Design review of the part built by this model. Coordinates are the model's own, in mm. A direction names the side the tool comes from. Give positions to 0.01 mm unless a question says otherwise; leave off trailing zeros. Order: outer loops, then holes, each group sorted by start corner. A loop starts at its lowest first (then second) coordinate and runs counter-clockwise, first axis right, second up. Notation, with made-up numbers: (55, 53.5) -> (104, 53.5) arc R14 cw to (104, 70.5) -> close; hole circle Ø4 at (22.25, 15). An arc over 180 degrees is marked (long way). One line per item, written item: value.
from build123d import *

# Parameters (mm, degrees)
SKETCH1_W            = 279.4
SKETCH1_H            = 101.6
BOSS_EXTRUDE1_DEPTH  = 6.35
SKETCH2_R            = 13.97
BOSS_EXTRUDE3_DEPTH  = 5.55625
SKETCH9_R            = 11.1125
CUT_EXTRUDE4_DEPTH   = 4.445
CUT_EXTRUDE5_START   = -5.55625
SKETCH10_R           = 11.1125
CUT_EXTRUDE5_DEPTH   = 5.55625
SKETCH11_R           = 7.9375
CUT_EXTRUDE6_DEPTH   = 285.078633923
SKETCH12_R           = 6.35
CUT_EXTRUDE7_DEPTH   = 285.051619429
SKETCH22_W           = 63.5
SKETCH22_H           = 63.5
BOSS_EXTRUDE7_DEPTH  = 12.7
SKETCH25_W           = 50.8
SKETCH25_H           = 50.8
CUT_EXTRUDE11_DEPTH  = 15.875
SKETCH32_R           = 4.7625
CUT_EXTRUDE12_DEPTH  = 6.35
SKETCH38_W           = 46.99
SKETCH38_H           = 18.470251096
CUT_EXTRUDE13_DEPTH  = 6.35
SKETCH60_R           = 4.7625
CUT_EXTRUDE23_DEPTH  = 6.35
SKETCH64_R           = 4.7625
CUT_EXTRUDE24_DEPTH  = 285.264471927
SKETCH65_W           = 52.07
SKETCH65_H           = 43.596758628
BOSS_EXTRUDE8_DEPTH  = 50.8
SKETCH68_W           = 43.596758628
SKETCH68_H           = 6.35
BOSS_EXTRUDE10_DEPTH = 6.35
SKETCH66_W           = 40.64
SKETCH66_H           = 32.500000024
CUT_EXTRUDE28_DEPTH  = 50.8
SKETCH69_W           = 40.64
SKETCH69_H           = 49.53
CUT_EXTRUDE29_DEPTH  = 292.497724665
SKETCH70_W           = 46.99
SKETCH70_H           = 2.529758466
CUT_EXTRUDE30_DEPTH  = 289.488543967


with BuildPart() as part:
    # Sketch1 → Boss-Extrude1 (new body)
    with BuildSketch(Plane(origin=(0, 0, 0), x_dir=(1, 0, 0), z_dir=(0, 1, 0))):
        with Locations((-139.7, 0)):
            Rectangle(SKETCH1_W, SKETCH1_H)
    extrude(amount=BOSS_EXTRUDE1_DEPTH)

    # Sketch2 → Boss-Extrude3 (add)
    with BuildSketch(Plane(origin=(0, 6.35, 0), x_dir=(1, 0, 0), z_dir=(0, 1, 0))):
        with Locations(Location((-258.510557857, 0, 0), (0, 0, 90))):
            Circle(SKETCH2_R)
    extrude(amount=BOSS_EXTRUDE3_DEPTH)

    # Sketch9 → Cut-Extrude4 (cut)
    with BuildSketch(Plane(origin=(0, 11.90625, 0), x_dir=(1, 0, 0), z_dir=(0, 1, 0))):
        with Locations(Location((-258.510557857, 0, 0), (0, 0, 270))):
            Circle(SKETCH9_R)
    extrude(amount=-CUT_EXTRUDE4_DEPTH, mode=Mode.SUBTRACT)

    # Sketch10 → Cut-Extrude5 (cut)
    with BuildSketch(Plane(origin=(0, 0, 0), x_dir=(-1, 0, 0), z_dir=(0, -1, 0)).offset(CUT_EXTRUDE5_START)):
        with Locations(Location((258.510557857, 0, 0), (0, 0, 270))):
            Circle(SKETCH10_R)
    extrude(amount=CUT_EXTRUDE5_DEPTH, mode=Mode.SUBTRACT)

    # Sketch11 → Cut-Extrude6 (cut, through all)
    with BuildSketch(Plane(origin=(0, 7.46125, 0), x_dir=(1, 0, 0), z_dir=(0, 1, 0))):
        with Locations(Location((-258.510557857, 0, 0), (0, 0, 270))):
            Circle(SKETCH11_R)
    extrude(amount=-CUT_EXTRUDE6_DEPTH, mode=Mode.SUBTRACT)

    # Sketch12 → Cut-Extrude7 (cut, through all)
    with BuildSketch(Plane(origin=(0, 6.35, 0), x_dir=(1, 0, 0), z_dir=(0, 1, 0))):
        with Locations(Location((-134.666203771, 0, 0), (0, 0, 270))):
            Circle(SKETCH12_R)
    extrude(amount=-CUT_EXTRUDE7_DEPTH, mode=Mode.SUBTRACT)

    # Sketch22 → Boss-Extrude7 (add)
    with BuildSketch(Plane(origin=(0, 6.35, 0), x_dir=(1, 0, 0), z_dir=(0, 1, 0))):
        with Locations((-134.666203771, 0)):
            Rectangle(SKETCH22_W, SKETCH22_H)
    extrude(amount=BOSS_EXTRUDE7_DEPTH)

    # Sketch25 → Cut-Extrude11 (cut)
    with BuildSketch(Plane(origin=(0, 19.05, 0), x_dir=(1, 0, 0), z_dir=(0, 1, 0))):
        with Locations((-134.666203771, 0)):
            Rectangle(SKETCH25_W, SKETCH25_H)
    extrude(amount=-CUT_EXTRUDE11_DEPTH, mode=Mode.SUBTRACT)

    # Sketch32 → Cut-Extrude12 (cut)
    with BuildSketch(Plane(origin=(0, 6.35, 0), x_dir=(1, 0, 0), z_dir=(0, 1, 0))):
        with Locations(Location((-67.44195898, -40.64, 0), (0, 0, 270))):
            Circle(SKETCH32_R)
        with Locations(Location((-81.41195898, -40.64, 0), (0, 0, 270))):
            Circle(SKETCH32_R)
        with Locations(Location((-67.44195898, 40.64, 0), (0, 0, 270))):
            Circle(SKETCH32_R)
        with Locations(Location((-81.41195898, 40.64, 0), (0, 0, 270))):
            Circle(SKETCH32_R)
    extrude(amount=-CUT_EXTRUDE12_DEPTH, mode=Mode.SUBTRACT)

    # Sketch38 → Cut-Extrude13 (cut)
    with BuildSketch(Plane(origin=(0, 6.35, 0), x_dir=(1, 0, 0), z_dir=(0, 1, 0))):
        with Locations((-23.495, -24.777709652)):
            Rectangle(SKETCH38_W, SKETCH38_H)
    extrude(amount=-CUT_EXTRUDE13_DEPTH, mode=Mode.SUBTRACT)

    # Sketch60 → Cut-Extrude23 (cut)
    with BuildSketch(Plane(origin=(0, 6.35, 0), x_dir=(1, 0, 0), z_dir=(0, 1, 0))):
        with Locations(Location((-231.7492444, 41.324145444, 0), (0, 0, 270))):
            Circle(SKETCH60_R)
        with Locations(Location((-231.7492444, -39.369341378, 0), (0, 0, 270))):
            Circle(SKETCH60_R)
        with Locations(Location((-173.509244294, -39.369341378, 0), (0, 0, 270))):
            Circle(SKETCH60_R)
        with Locations(Location((-173.509244294, 41.324145444, 0), (0, 0, 270))):
            Circle(SKETCH60_R)
    extrude(amount=-CUT_EXTRUDE23_DEPTH, mode=Mode.SUBTRACT)

    # Sketch64 → Cut-Extrude24 (cut, through all)
    with BuildSketch(Plane(origin=(0, 6.35, 0), x_dir=(1, 0, 0), z_dir=(0, 1, 0))):
        with Locations(Location((-145.334203771, -41.275, 0), (0, 0, 270))):
            Circle(SKETCH64_R)
        with Locations(Location((-123.998203771, -41.275, 0), (0, 0, 270))):
            Circle(SKETCH64_R)
    cut_extrude24 = extrude(amount=-CUT_EXTRUDE24_DEPTH, mode=Mode.SUBTRACT)

    # Mirror1: Cut-Extrude24 across plane
    add(cut_extrude24.mirror(Plane.XY), mode=Mode.SUBTRACT)

    # Sketch65 → Boss-Extrude8 (add)
    with BuildSketch(Plane(origin=(0, 6.35, 0), x_dir=(1, 0, 0), z_dir=(0, 1, 0))):
        with Locations((-19.685, 8.785553676)):
            Rectangle(SKETCH65_W, SKETCH65_H)
    extrude(amount=BOSS_EXTRUDE8_DEPTH)

    # Sketch68 → Boss-Extrude10 (add)
    with BuildSketch(Plane(origin=(0, 0, 0), x_dir=(0, 0, -1), z_dir=(1, 0, 0))):
        with Locations((8.785553676, 3.175)):
            Rectangle(SKETCH68_W, SKETCH68_H)
    extrude(amount=BOSS_EXTRUDE10_DEPTH)

    # Sketch66 → Cut-Extrude28 (cut)
    with BuildSketch(Plane(origin=(0, 57.15, 0), x_dir=(1, 0, 0), z_dir=(0, 1, 0))):
        with Locations((-20.32, 6.713932978)):
            Rectangle(SKETCH66_W, SKETCH66_H)
    extrude(amount=-CUT_EXTRUDE28_DEPTH, mode=Mode.SUBTRACT)

    # Sketch69 → Cut-Extrude29 (cut, through all)
    with BuildSketch(Plane(origin=(0, 0, 9.536067034), x_dir=(-1, 0, 0), z_dir=(0, 0, -1))):
        with Locations((20.32, 32.385)):
            Rectangle(SKETCH69_W, SKETCH69_H)
    extrude(amount=-CUT_EXTRUDE29_DEPTH, mode=Mode.SUBTRACT)

    # Sketch70 → Cut-Extrude30 (cut, through all)
    with BuildSketch(Plane(origin=(0, 6.35, 0), x_dir=(1, 0, 0), z_dir=(0, 1, 0))):
        with Locations((-23.495, -14.277704871)):
            Rectangle(SKETCH70_W, SKETCH70_H)
    extrude(amount=-CUT_EXTRUDE30_DEPTH, mode=Mode.SUBTRACT)


solid = part.part
Item 1: Add section D-D on z = 21. Give the boundary of the cut face in (x, y) (3 decimals).
Returned:
outline: (-279.4, 0) -> (-46.99, 0) -> (-46.99, 6.35) -> (-102.916, 6.35) -> (-102.916, 19.05) -> (-109.266, 19.05) -> (-109.266, 3.175) -> (-160.066, 3.175) -> (-160.066, 19.05) -> (-166.416, 19.05) -> (-166.416, 6.35) -> (-279.4, 6.35) -> close
Item 2: Machinability: for faces 1 (the flat face through (-24, 3, 34.013)), 2 (the flat face through (-135, 11, -25.4)), 3 (the flat face through (0, 3, 43)), 4 (the cylindrical face through (-72.09, 3.22, -41.67)), 5 (the flat face through (-20, 57.15, -24)), which of the approach directions +Z, -Z, +X, -X, +Y, -Y give a long, thin tool a straight path to every point of the face, cutting with its end or side? Answer none if there is none.
Returned:
face 1: +X, +Y, -Y
face 2: +Y
face 3: +Z, +X, +Y, -Y
face 4: +Y, -Y
face 5: +Z, -Z, +X, -X, +Y
Item 3: Add section A-A on x = -13.5. Give the boundary of the cut face in (y, z), plus the area to 3 significant figures.
Returned:
outline: (0, -50.8) -> (6.35, -50.8) -> (6.35, -30.58) -> (57.15, -30.58) -> (57.15, -22.96) -> (6.35, -22.96) -> (6.35, 9.54) -> (7.62, 9.54) -> (7.62, 13.01) -> (0, 13.01) -> close; (0, 34.01) -> (6.35, 34.01) -> (6.35, 50.8) -> (0, 50.8) -> close
area: 903 mm²
Item 4: To check wall thickness, follow line 1 along X through (y, z) = (7.5, -15); line 2 along X through (y, z) = (27.5, 3.5); line 3 along Z through (x, y) = (-258.5, 5). State the ranges of each line that lie inside material, in increasing order. Write a range as from..to.
Returned:
line 1: -166.42..-160.07, -109.27..-102.92, -45.72..-40.64, 0..6.35
line 2: -45.72..-40.64, 0..6.35
line 3: -50.8..-11.11, 11.11..50.8
Item 5: Add section C-C on z = 40.64. Give the boundary of the cut face in (x, y).
Returned:
outline: (-279.4, 0) -> (-236.34, 0) -> (-236.34, 6.35) -> (-279.4, 6.35) -> close; (-227.16, 0) -> (-178.1, 0) -> (-178.1, 6.35) -> (-227.16, 6.35) -> close; (-168.92, 0) -> (-150.05, 0) -> (-150.05, 6.35) -> (-168.92, 6.35) -> close; (-140.61, 0) -> (-128.72, 0) -> (-128.72, 6.35) -> (-140.61, 6.35) -> close; (-119.28, 0) -> (-86.17, 0) -> (-86.17, 6.35) -> (-119.28, 6.35) -> close; (-76.65, 0) -> (-72.2, 0) -> (-72.2, 6.35) -> (-76.65, 6.35) -> close; (-62.68, 0) -> (0, 0) -> (0, 6.35) -> (-62.68, 6.35) -> close
Item 6: Clearance check with flat-ended pins moving along their axes: P1, Ø12.5, axis at x = -231.75, z = 39.37, coming from the +Y side; P2, Ø7, axis at y = 1.5, z = 26, coming from the +X side; P3, Ø3, axis at y = 42, z = -7, coming from the -X side. State where each tip first meets the part, or that it passes through.
Returned:
P1: y = 6.35
P2: x = -46.99
P3: x = -45.72
Item 7: Add section B-B on y = 53.5. Give the boundary of the cut face in (x, z), plus the area to 3 significant figures.
Returned:
outline: (-45.72, -30.58) -> (6.35, -30.58) -> (6.35, 13.01) -> (0, 13.01) -> (0, -22.96) -> (-40.64, -22.96) -> (-40.64, 13.01) -> (-45.72, 13.01) -> close
area: 808 mm²
